Part model, mm, in its own coordinate system. A direction names the side the tool comes from. Coordinates: 2 decimals unless noted, no trailing zeros. Order: outer loops, then holes, each group sorted by start corner. A loop starts at its lowest first (then second) coordinate and runs counter-clockwise, first axis right, second up.
1) Wall check: L1, parallel to Y at x = 81.5, z = 84.5; L2, parallel to X at y = 17, z = 73; L3, parallel to Z at x = 60, y = 107.5. Give the ranges that are in metal, low to high.
2) Mould opens along Y. For faces 1 (the cylindrical face through (60.2, 144.2, 3.2)), 2 (the flat face through (45, 0, 51)), 3 (the flat face through (46, 1.5, 42)) say: +Y half, -Y half, draft (parallel to the pull), parting line (faces both ways), or undercut.
3) Pin check, flat tips, straight feed: pin 1 Ø1.2 at (x, z) = (0.5, 25) entering from +Y; pin 2 Ø11.5 at (y, z) = (-6, -1.5) entering from -X; pin 3 Ø0.8 at (x, y) = (90.5, 55) entering from -Z. Stop position of each tip, or through.
4) Cut at A-A (z = 43.5). List the corners of the cut face in (x, y), and give its area (3 significant figures).
5) Cut at B-B (y = 127). List the corners of the cut face in (x, z).
6) Tool access for faces 4 (the flat face through (2, -2, -3)), 5 (the flat face through (90.1, 70, 47)), 6 (the flat face through (60, 150.4, -5)), 7 (the flat face through (30, 143.7, 3.5)), 8 (the flat face through (45, 141.6, 51)): list every direction of +Z, -Z, +X, -X, +Y, -Y with a clear straight run to the whole face (end or side of a thin tool).
7) Cut at C-C (x = 53). List the corners of the cut face in (y, z), and give its area (3 significant figures).
```python
from build123d import *

# Parameters (mm, degrees)
SKETCH1_W             = 141.6
SKETCH1_H             = 94.4
BOSS_EXTRUDE1_DEPTH   = 91.6
SHELL1_T              = -1.5
SKETCH2_W             = 141.6
SKETCH2_H             = 14
CUT_EXTRUDE1_DEPTH    = 2
SKETCH3_W             = 30
SKETCH3_H             = 37
CUT_EXTRUDE2_DEPTH    = 2
SKETCH4_W             = 91.6
SKETCH4_H             = 8.8
BOSS_EXTRUDE2_DEPTH   = 9.5
SKETCH4_W_2           = 61.6
BOSS_EXTRUDE2_2_DEPTH = 9.5
SKETCH5_W             = 91.6
SKETCH5_H             = 1.5
SKETCH5_W_2           = 61.6
BOSS_EXTRUDE3_DEPTH   = 9.5
FILLET1_R             = 10
SKETCH6_W             = 2
SKETCH6_H             = 10.3
CUT_EXTRUDE3_DEPTH    = 200.80510504
FILLET2_R             = 2


with BuildPart() as part:
    # Sketch1 → Boss-Extrude1 (new body)
    with BuildSketch(Plane.YZ):
        with Locations((70.8, 47.2)):
            Rectangle(SKETCH1_W, SKETCH1_H)
    extrude(amount=BOSS_EXTRUDE1_DEPTH)

    # Shell1
    shell1_openings = [part.faces().sort_by_distance(p)[0] for p in [
        (45.8, 70.8, 0),
    ]]
    offset(amount=SHELL1_T, openings=shell1_openings, kind=Kind.INTERSECTION)

    # Sketch2 → Cut-Extrude1 (cut)
    with BuildSketch(Plane(origin=(0, 0, 0), x_dir=(0, -1, 0), z_dir=(-1, 0, 0))):
        with Locations((-70.8, 7)):
            Rectangle(SKETCH2_W, SKETCH2_H)
    extrude(amount=-CUT_EXTRUDE1_DEPTH, mode=Mode.SUBTRACT)

    # Sketch3 → Cut-Extrude2 (cut)
    with BuildSketch(Plane(origin=(0, 141.6, 0), x_dir=(1, 0, 0), z_dir=(0, 1, 0))):
        with Locations((15, -18.5)):
            Rectangle(SKETCH3_W, SKETCH3_H)
    extrude(amount=-CUT_EXTRUDE2_DEPTH, mode=Mode.SUBTRACT)



with BuildPart() as body_2:
    # Sketch4 → Boss-Extrude2 (new body)
    with BuildSketch(Plane(origin=(0, 0, 0), x_dir=(1, 0, 0), z_dir=(0, 0, -1))):
        with Locations((45.8, 4.4)):
            Rectangle(SKETCH4_W, SKETCH4_H)
    extrude(amount=BOSS_EXTRUDE2_DEPTH)


with BuildPart() as body_3:
    # Sketch4 → Boss-Extrude2 2 (new body)
    with BuildSketch(Plane(origin=(0, 0, 0), x_dir=(1, 0, 0), z_dir=(0, 0, -1))):
        with Locations((60.8, -146)):
            Rectangle(SKETCH4_W_2, SKETCH4_H)
    extrude(amount=BOSS_EXTRUDE2_2_DEPTH)


with BuildPart() as part_1:
    add(part.part)

    add(body_2.part)  # Boss-Extrude3 merges body 2

    add(body_3.part)  # Boss-Extrude3 merges body 3
    # Sketch5 → Boss-Extrude3 (add)
    with BuildSketch(Plane(origin=(0, 0, 0), x_dir=(1, 0, 0), z_dir=(0, 0, -1))):
        with Locations((45.8, -0.75)):
            Rectangle(SKETCH5_W, SKETCH5_H)
        with Locations((60.8, -140.85)):
            Rectangle(SKETCH5_W_2, SKETCH5_H)
    extrude(amount=BOSS_EXTRUDE3_DEPTH)

    # Fillet1
    # the kernel refuses this fillet: 10 mm, written as the material it adds along each edge
    with BuildSketch(Plane(origin=(91.6, 0, 0), x_dir=(0, 0, 1), z_dir=(-1, 0, 0))) as fillet1_piece_1:
        with BuildLine():
            CenterArc((9.927738917, -10), FILLET1_R, 90, 83.107897421)
            Line((0, -8.8), (-0.198554778, -8.776))
            ThreePointArc((-0.198554778, -8.776), (-0.2, -4.4), (-0.2, 0))
            Line((-0.2, 0), (0, 0.2))
            Line((0, 0.2), (9.927738917, 0.2))
            Line((9.927738917, 0.2), (9.927738917, 0))
        make_face()
    extrude(amount=89.6)
    with BuildSketch(Plane(origin=(91.6, 141.6, 0), x_dir=(0, 0, 1), z_dir=(-1, 0, 0))) as fillet1_piece_2:
        with BuildLine():
            CenterArc((9.927738917, 10), FILLET1_R, 186.892102579, 83.107897421)
            Line((0, 8.8), (-0.198554778, 8.776))
            ThreePointArc((-0.198554778, 8.776), (-0.2, 4.4), (-0.2, 0))
            Line((-0.2, 0), (0, -0.2))
            Line((0, -0.2), (9.927738917, -0.2))
            Line((9.927738917, -0.2), (9.927738917, 0))
        make_face()
    extrude(amount=61.6)

    # Sketch6 → Cut-Extrude3 (cut, through all)
    with BuildSketch(Plane.XY):
        with Locations((1, -3.65)):
            Rectangle(SKETCH6_W, SKETCH6_H)
    extrude(amount=-CUT_EXTRUDE3_DEPTH, mode=Mode.SUBTRACT)

    # Fillet2
    fillet2_edges = [part_1.edges().sort_by_distance(p)[0] for p in [
        (91.6, 144.116685226, 3.294489336),
        (91.6, -2.516685226, 3.294489336),
        (0, 0, 54.2),
        (0, 141.6, 65.7),
        (91.6, 141.6, 52.163869458),
        (91.6, 0, 52.163869458),
        (0, 70.8, 94.4),
        (45.8, 0, 94.4),
        (91.6, 70.8, 94.4),
        (45.8, 141.6, 94.4),
    ]]
    fillet(fillet2_edges, radius=FILLET2_R)


solid = part_1.part
```
Geometry check:
1. L1: y = 0 to 1.5, 140.1 to 141.6
1. L2: x = 0 to 1.5, 90.1 to 91.6
1. L3: z = 92.9 to 94.4
2. face 1: +Y half
2. face 2: -Y half
2. face 3: undercut
3. pin 1: stops at y = 139.6
3. pin 2: stops at x = 2
3. pin 3: stops at z = 0
4. outline: (0, 2) arc R2 ccw to (2, 0) - (89.6, 0) arc R2 ccw to (91.6, 2) - (91.6, 139.6) arc R2 ccw to (89.6, 141.6) - (2, 141.6) arc R2 ccw to (0, 139.6) - close; hole (1.5, 1.5) - (90.1, 1.5) - (90.1, 140.1) - (1.5, 140.1) - close
4. area: 687 mm2
5. outline: (0, 14) - (1.5, 14) - (1.5, 92.9) - (90.1, 92.9) - (90.1, 0) - (91.6, 0) - (91.6, 92.4) arc R2 ccw to (89.6, 94.4) - (2, 94.4) arc R2 ccw to (0, 92.4) - close
6. face 4: -Z, -X, +Y, -Y
6. face 5: -Z
6. face 6: +Z, -Z, +X, -X, +Y
6. face 7: -Z, -X, +Y
6. face 8: +Z, +X, -X, +Y
7. outline: (-8.8, -9.5) - (1.5, -9.5) - (1.5, 92.9) - (140.1, 92.9) - (140.1, -9.5) - (150.4, -9.5) - (150.4, 0) arc R10 cw to (141.6, 9.93) - (141.6, 92.4) arc R2 ccw to (139.6, 94.4) - (2, 94.4) arc R2 ccw to (0, 92.4) - (0, 9.93) arc R10 cw to (-8.8, 0) - close
7. area: 727 mm2
